Autodesk Fusion 360 part; units mm, degrees
sketch "Sketch1" plane through (0, 0, 0) normal (0, 0, 1) x (1, 0, 0)
  line L0 (-10, 22.5) -> (10, 22.5)
  line L1 (10, 22.5) -> (10, -22.5)
  line L2 (10, -22.5) -> (-10, -22.5)
  line L3 (-10, -22.5) -> (-10, 22.5)
  line L4 (10, 12.5) -> (5, 12.5)
  line L5 (5, 12.5) -> (5, -12.5)
  line L6 (5, -12.5) -> (10, -12.5)
  line L7 (10, -12.5) -> (10, 12.5)
  line L8 (0, 22.5) -> (0, -22.5)
  line L9 (-10, 22.5) -> (-10, -22.5)
  line L10 (-10, -12.5) -> (-10, 12.5)
  line L11 (-5, -12.5) -> (-10, -12.5)
  line L12 (-5, 12.5) -> (-5, -12.5)
  line L13 (-10, 0) -> (10, 0)
  line L14 (-10, 12.5) -> (10, 12.5)
  line L15 (10, 12.5) -> (10, 5)
  line L16 (10, 5) -> (-10, 5)
  line L17 (-10, 5) -> (-10, 12.5)
  line L18 (10, -5) -> (-10, -5)
  line L19 (-10, -12.5) -> (10, -12.5)
  dimension "d1" = 20
  dimension "d2" = 45
  dimension "d3" = 22.5
  dimension "d4" = 10
  dimension "d5" = 5
  dimension "d6" = 25
  dimension "d7" = 12.5
  dimension "d8" = 7.5
  dimension "d9" = 10
extrude "Extrude1" add sketch "Sketch1" along normal blind 25 contours L3 L9 L10 L12 L14 L16 L17 | L5 L8 L14 L16 | L8 L12 L14 L16 | L1 L4 L5 L7 L14 L15 L16 | L3 L9 L10 L11 L12 L18 L19 | L5 L8 L18 L19 | L8 L12 L18 L19 | L1 L5 L6 L7 L18 L19 makes body 1 at (-3.3333, 12.5, 8.3333) makes body 2 at (3.3333, -5, 8.3333)
extrude "Extrude2" add sketch "Sketch1" against normal blind 25 contours L3 L9 L10 L12 L14 L16 L17 | L3 L9 L10 L12 L13 L16 | L1 L4 L5 L7 L14 L15 L16 | L3 L9 L10 L12 L13 L18 | L1 L5 L7 L13 L16 | L3 L9 L10 L11 L12 L18 L19 | L1 L5 L7 L13 L18 | L1 L5 L6 L7 L18 L19 bodies 1 2
extrude "Extrude3" add sketch "Sketch1" along normal blind 5 contours L0 L3 L8 L9 L14 | L0 L1 L4 L8 L14 | L3 L9 L10 L12 L13 L16 | L5 L8 L13 L16 | L8 L12 L13 L16 | L3 L9 L10 L12 L13 L18 | L1 L5 L7 L13 L16 | L5 L8 L13 L18 | L8 L12 L13 L18 | L1 L5 L7 L13 L18 | L2 L3 L8 L9 L11 L19 | L1 L2 L6 L8 L19 bodies 1
fillet "Fillet1" radius 12.5 4 edges at (7.5, -12.5, -25) (-7.5, -12.5, -25) (-7.5, 12.5, -25) (7.5, 12.5, -25) on bodies 1
fillet "Fillet2" radius 2 2 edges at (0, -5, 5) (0, 5, 5) on bodies 1
sketch "Sketch2" plane through (10, 0, 0) normal (1, 0, 0) x (0, 1, 0)
  arc A0 (-12.5, -12.5) -> (12.5, -12.5) centre (0, -12.5) ccw
  line L0 (12.5, -12.5) -> (12.5, 0)
  line L1 (12.5, 0) -> (22.5, 0)
  line L2 (22.5, 0) -> (22.5, 5)
  line L3 (22.5, 5) -> (12.5, 5)
  line L4 (12.5, 5) -> (12.5, 25)
  line L5 (12.5, 25) -> (5, 25)
  line L6 (5, 25) -> (5, 7)
  arc A1 (3, 5) -> (5, 7) centre (3, 7) ccw
  line L7 (3, 5) -> (-3, 5)
  arc A2 (-5, 7) -> (-3, 5) centre (-3, 7) ccw
  line L8 (-5, 7) -> (-5, 25)
  line L9 (-5, 25) -> (-12.5, 25)
  line L10 (-12.5, 25) -> (-12.5, 5)
  line L11 (-12.5, 5) -> (-22.5, 5)
  line L12 (-22.5, 5) -> (-22.5, 0)
  line L13 (-22.5, 0) -> (-12.5, 0)
  line L14 (-12.5, 0) -> (-12.5, -12.5)
  circle A3 centre (0, -12.5) radius 6.25
  dimension "d20" = 12.5
  dimension "d21" = 12.5
extrude "Extrude4" cut sketch "Sketch2" against normal up to surface (20 mm away) contours A3 bodies 1
equation "d3 = ( 45 / 2 ) * 1 mm"
equation "d7 = ( 25 / 2 ) * 1 mm"
equation "d8 = ( 15 / 2 ) * 1 mm"
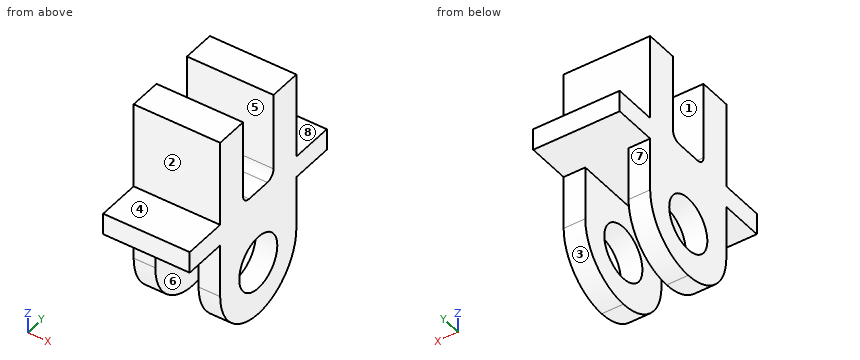
Verification items for the finished model (mm, model axes). Face numbers are marked on the shaded views. A direction names the side the tool comes from. Give positions to 0.01 mm unless a question says otherwise; leave off trailing zeros. Order: outer loops, then holes, each group sorted by start corner. A loop starts at its lowest first (then second) coordinate and runs counter-clockwise, first axis right, second up. Notation, with made-up numbers: M 58.5,71 L 109.5,71 A14 cw 109.5,80 Z; hole C 88.25,2.25 d1. An arc over 180 degrees is marked long. Answer as a JSON object with one key per item and string values. Group by question number.
1) Cross-section at D-D (x = 4.25). Enter the section's corners in (y, z).
2) Cross-section at A-A (z = -7). Enter the section's corners in (x, y), then the cut area to 3 significant figures.
3) Cross-section at C-C (y = 10). Enter the section's corners in (x, z).
4) Depth check by flat-ended pin: pin 1 Ø6.5 at (x, y) = (3, -0.5) entering from +Z; pin 2 Ø10 at (x, z) = (-2, 16.5) entering from -Y; pin 3 Ø3 at (x, y) = (-3.5, -14) entering from -Z. Enter the tip coordinate at first touch or a pass-through.
5) Access from +Z, -Z, +X, -X, +Y, -Y to the whole of each face (thin tool, end or side, straight path). Record for the marked faces 4, 5, 6, 7 and 8.
6) Mould release check, pull along Y, two halves, no side actions. Record for the marked faces 1, 2 and 3: released by +Y, released by -Y, zero draft, split by the parting line, or undercut.
7) Scan lines: line 1 along Y through (x, z) = (-0.75, 19); line 2 along Z through (x, y) = (7.4, 0); line 3 along X through (y, z) = (5, -3). Record each from-to range of solid material in increasing order. Write a range as [from, to].
Result sheet:
{
 "1": {"outline": "M -22.5,0 L 22.5,0 L 22.5,5 L 12.5,5 L 12.5,25 L 5,25 L 5,7 A2 cw 3,5 L -3,5 A2 cw -5,7 L -5,25 L -12.5,25 L -12.5,5 L -22.5,5 Z"},
 "2": {"outline": "M -10,-12.5 L -5,-12.5 L -5,-2.97 L -10,-2.97 Z; M -10,2.97 L -5,2.97 L -5,12.5 L -10,12.5 Z; M 5,-12.5 L 10,-12.5 L 10,-2.97 L 5,-2.97 Z; M 5,2.97 L 10,2.97 L 10,12.5 L 5,12.5 Z", "area": "191 mm2"},
 "3": {"outline": "M -10,-20 L -5,-20 L -5,0 L 5,0 L 5,-20 L 10,-20 L 10,25 L -10,25 Z"},
 "4": {"pin 1": "stops at z = 5.15", "pin 2": "stops at y = -12.5", "pin 3": "stops at z = 0"},
 "5": {"face 4": "+Z, +X, -X, -Y", "face 5": "+Z, +X, -X", "face 6": "-Z, +Y, -Y", "face 7": "-Z, +X, -X, +Y", "face 8": "+Z, +X, -X, +Y"},
 "6": {"face 1": "undercut", "face 2": "released by -Y", "face 3": "released by +Y"},
 "7": {"line 1": "y = [-12.5, -5], [5, 12.5]", "line 2": "z = [-25, -18.75], [-6.25, 5]", "line 3": "x = [-10, -5], [5, 10]"}
}
